```python
from build123d import *

# Parameters (mm, degrees)
BOSS_EXTRUDE1_DEPTH = 12.7
CUT_EXTRUDE1_DEPTH  = 6.35
BOSS_EXTRUDE2_DEPTH = 6.35


with BuildPart() as part:
    # Sketch1 → Boss-Extrude1 (new body)
    with BuildSketch(Plane(origin=(0, 0, 0), x_dir=(1, 0, 0), z_dir=(0, 1, 0))):
        with BuildLine():
            Line((-33.655, -40.005), (33.655, -40.005))
            ThreePointArc((33.655, -40.005), (38.145128061, -38.145128061), (40.005, -33.655))
            Line((40.005, -33.655), (40.005, 33.655))
            ThreePointArc((40.005, 33.655), (38.145128061, 38.145128061), (33.655, 40.005))
            Line((33.655, 40.005), (-33.655, 40.005))
            ThreePointArc((-33.655, 40.005), (-38.145128061, 38.145128061), (-40.005, 33.655))
            Line((-40.005, 33.655), (-40.005, -33.655))
            ThreePointArc((-40.005, -33.655), (-38.145128061, -38.145128061), (-33.655, -40.005))
        make_face()
    extrude(amount=BOSS_EXTRUDE1_DEPTH)

    # Sketch2 → Cut-Extrude1 (cut)
    with BuildSketch(Plane(origin=(0, 12.7, 0), x_dir=(1, 0, 0), z_dir=(0, 1, 0))):
        with BuildLine():
            Line((-40.005, 3.81), (-37.321374038, 9.565054448))
            ThreePointArc((-37.321374038, 9.565054448), (-29.576722684, 0), (-37.321374038, -9.565054448))
            Line((-37.321374038, -9.565054448), (-40.005, -3.81))
            Line((-40.005, -3.81), (-40.005, 3.81))
        make_face()
    extrude(amount=-CUT_EXTRUDE1_DEPTH, mode=Mode.SUBTRACT)

    # Sketch4 → Boss-Extrude2 (add)
    with BuildSketch(Plane(origin=(0, 12.7, 0), x_dir=(1, 0, 0), z_dir=(0, 1, 0))):
        with BuildLine():
            Line((42.688625962, 9.565054448), (40.005, 3.81))
            Line((40.005, 3.81), (40.005, -3.81))
            Line((40.005, -3.81), (42.688625962, -9.565054448))
            ThreePointArc((42.688625962, -9.565054448), (50.433277316, 0), (42.688625962, 9.565054448))
        make_face()
    extrude(amount=-BOSS_EXTRUDE2_DEPTH)


solid = part.part
```
Check sheet for the modelled part. Datum: model origin and axes. Units: mm. A direction names the side the tool comes from. Round coordinates to 2 decimals unless told otherwise and drop trailing zeros. Order: outer loops, then holes, each group sorted by start corner. A loop starts at its lowest first (then second) coordinate and runs counter-clockwise, first axis right, second up.
1) Mould release check, pull along X, two halves, no side actions. Record for faces 4 (the cylindrical face through (38.19, 6.26, -38.1)), 5 (the flat face through (-1, 0, -1)), 6 (the flat face through (41.366, 9.569, -6.728)): +X half, -X half, draft (parallel to the pull), parting line (faces both ways), or undercut.
2) Go/stop test with flat-tipped pins: pin 1 Ø5 at (y, z) = (3, 26) entering from +X (3 decimals); pin 2 Ø4 at (y, z) = (8, -7.5) entering from +X; pin 3 Ø5 at (x, z) = (47.5, 1) entering from -Y. Record where each tip stops, or that it passes through.
3) Section check B-B (z = -6.5). Record the boundary of the cut face in (x, y) (3 decimals).
4) Scan lines: line 1 (X direction, y = 3, z = 30) (3 decimals); line 2 (X direction, y = 7, z = 1); line 3 (Z direction, x = 34.5, y = 12.25). Record each from-to range of solid material in increasing order.
5) Tool access check on faces 1 (the flat face through (0, 6, 40.005)), 2 (the flat face through (-38.644, 9.569, 6.728)), 3 (the flat face through (45, 6.35, 0)). Record the directions out of +Z, -Z, +X, -X, +Y, -Y that give a thin tool (end or side, any length) a straight path to the whole face; none if there is none.
6) Section check A-A (y = 9.5). Record the boundary of the cut face in (x, z) (3 decimals), and give its area (3 significant figures).
7) Section check C-C (z = 27.5). Record the boundary of the cut face in (x, y) (3 decimals).
Result:
1. face 4: +X half
1. face 5: draft
1. face 6: undercut
2. pin 1: stops at x = 40.005
2. pin 2: stops at x = 48.74
2. pin 3: stops at y = 6.35
3. outline: (-40.005, 0) - (40.005, 0) - (40.005, 12.7) - (-32.05, 12.7) - (-32.05, 6.35) - (-38.751, 6.35) - (-38.751, 12.7) - (-40.005, 12.7) - close; (41.259, 6.35) - (47.96, 6.35) - (47.96, 12.7) - (41.259, 12.7) - close
4. line 1: x = -40.005 to 40.005
4. line 2: x = -29.63 to 50.38
4. line 3: z = -39.95 to 39.95
5. face 1: +Z, +X, -X, +Y, -Y
5. face 2: +Y
5. face 3: +Z, -Z, +X, -Y
6. outline: (-40.005, -33.655) arc R6.35 ccw to (-33.655, -40.005) - (33.655, -40.005) arc R6.35 ccw to (40.005, -33.655) - (40.005, -3.81) - (42.689, -9.565) arc R9.779 ccw to (42.689, 9.565) - (40.005, 3.81) - (40.005, 33.655) arc R6.35 ccw to (33.655, 40.005) - (-33.655, 40.005) arc R6.35 ccw to (-40.005, 33.655) - (-40.005, 3.81) - (-37.321, 9.565) arc R9.779 cw to (-37.321, -9.565) - (-40.005, -3.81) - close
6. area: 6,370 mm2
7. outline: (-40.005, 0) - (40.005, 0) - (40.005, 12.7) - (-40.005, 12.7) - close
